Input: part model. Units: mm. Frame: model coordinates. Face numbers are marked on the shaded views. A direction names the side the tool comes from. Round coordinates to 2 decimals unless told otherwise and drop trailing zeros. Order: outer loops, then holes, each group sorted by start corner. A loop starts at its lowest first (then second) coordinate and runs counter-clockwise, first axis right, second up.
Item 1: Cut plane B-B on y = 13. Output: boundary loops of the cut face in (x, z).
Item 2: Cut plane A-A on x = -3. Output: boundary loops of the cut face in (y, z), then the cut area to 3 significant figures.
Item 3: Line query: L1, parallel to Y at x = -22.5, z = -3.35; L2, parallel to Z at x = -17, y = 29; L3, parallel to Y at x = -7, z = -19.25. Output: solid intervals per line, ascending.
Item 4: Cut plane C-C on x = -22.5. Output: boundary loops of the cut face in (y, z).
Item 5: Mould query, pull axis Y, two halves, no side actions, for the marked faces 3, 4 and 5. Classes: released by +Y, released by -Y, zero draft, split by the parting line, or undercut.
Item 6: Reachability of the marked faces 1 and 2 from +Z, -Z, +X, -X, +Y, -Y: full face, straight path, thin tool, end or side. Return the list, or none.
Item 7: First-contact query: pin 1 (3 mm diameter, centred on y = 19.5, z = -4, fed in from +X); pin 2 (8 mm diameter, centred on y = 13, z = -12, fed in from +X). Flat tips, straight axial feed; report the tip coordinate or a pass-through.
Item 8: Cut plane D-D on y = 22. Output: boundary loops of the cut face in (x, z).
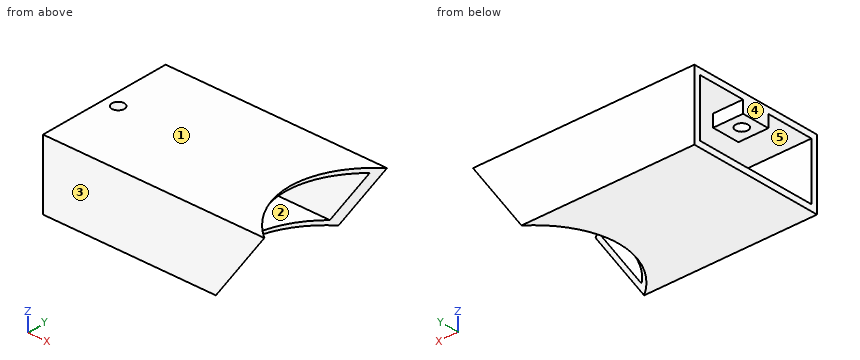
```python
from build123d import *

# Parameters (mm, degrees)
BOSS_EXTRUDE1_DEPTH      = 60
BOSS_EXTRUDE1_DEPTH_BACK = 27
SKETCH1_W                = 22.45
SKETCH1_H                = 43.9
SKETCH1_W_2              = 18.45
SKETCH1_H_2              = 39.9
SKETCH3_W                = 9.697753833
SKETCH3_H                = 9.057928037
SKETCH3_R                = 2
BOSS_EXTRUDE2_DEPTH      = 6
CUT_EXTRUDE1_REACH       = 66.258
SKETCH3_3_R              = 2


with BuildPart() as part:
    # Sketch1 → Boss-Extrude1 (new, two sides: drawn at the far end of the back side and taken through both)
    with BuildSketch(Plane(origin=(0, 0, 0), x_dir=(0, 0, -1), z_dir=(1, 0, 0)).offset(-BOSS_EXTRUDE1_DEPTH_BACK)):
        with Locations((10.58634259, 18.324330998)):
            Rectangle(SKETCH1_W, SKETCH1_H)
        with Locations((10.58634259, 18.324330998)):
            Rectangle(SKETCH1_W_2, SKETCH1_H_2, mode=Mode.SUBTRACT)
    extrude(amount=BOSS_EXTRUDE1_DEPTH + BOSS_EXTRUDE1_DEPTH_BACK)

    # Sketch2 → Cut-Revolve1 (revolve, cut)
    with BuildSketch(Plane(origin=(0, 18.324330998, 0), x_dir=(-1, 0, 0), z_dir=(0, -1, 0))):
        Polygon((-79.85393198, -15.110595304), (-55.279370652, -32.317888394), (-13.19002891, 27.791921119), (-37.764590239, 44.999214209), align=None)
    revolve(axis=Axis((79.85393198, 18.324330998, 15.110595304), (-0.573576436351041, 0, -0.8191520442889954)), mode=Mode.SUBTRACT)

    # Sketch3 → Boss-Extrude2 (add)
    with BuildSketch(Plane.XY.offset(0.63865741)):
        with Locations((-22.151123083, 18.324330997)):
            Rectangle(SKETCH3_W, SKETCH3_H)
        with Locations((-22.5, 18.324330998)):
            Circle(SKETCH3_R, mode=Mode.SUBTRACT)
    extrude(amount=-BOSS_EXTRUDE2_DEPTH)

    # Sketch3<3> → Cut-Extrude1 (cut, up to next)
    with BuildSketch(Plane.XY.offset(0.63865741), mode=Mode.PRIVATE) as cut_extrude1_sk1:
        with Locations((-22.5, 18.324330998)):
            Circle(SKETCH3_3_R)
    cut_extrude1_tool1 = extrude(cut_extrude1_sk1.sketch, amount=-CUT_EXTRUDE1_REACH, mode=Mode.PRIVATE) & part.part
    add(cut_extrude1_tool1.solids().sort_by_distance((-22.5, 18.324331, 0.638657))[0], mode=Mode.SUBTRACT)


solid = part.part
```
From the geometry:
1. outline: (-27, -21.81) - (17.96, -21.81) - (19.36, -19.81) - (-27, -19.81) - close; (-27, -1.36) - (32.28, -1.36) - (33.68, 0.64) - (-27, 0.64) - close
2. outline: (-3.63, -21.81) - (40.27, -21.81) - (40.27, 0.64) - (-3.63, 0.64) - close; hole (-1.63, -19.81) - (38.27, -19.81) - (38.27, -1.36) - (-1.63, -1.36) - close
2. area: 249 mm2
3. L1: y = -3.63 to -1.63, 13.8 to 16.32, 20.32 to 22.85, 38.27 to 40.27
3. L2: z = -21.81 to -19.81, -1.36 to 0.64
3. L3: y = -3.63 to -1.63, 38.27 to 40.27
4. outline: (-3.63, -21.81) - (40.27, -21.81) - (40.27, 0.64) - (20.32, 0.64) - (20.32, -5.36) - (22.85, -5.36) - (22.85, -1.36) - (38.27, -1.36) - (38.27, -19.81) - (-1.63, -19.81) - (-1.63, -1.36) - (13.8, -1.36) - (13.8, -5.36) - (16.32, -5.36) - (16.32, 0.64) - (-3.63, 0.64) - close
5. face 3: released by -Y
5. face 4: zero draft
5. face 5: undercut
6. face 1: +Z, +X, -X, +Y, -Y
6. face 2: +X, -X
7. pin 1: stops at x = -17.3
7. pin 2: passes through
8. outline: (-27, -21.81) - (17.65, -21.81) - (19.05, -19.81) - (-27, -19.81) - close; (-27, -5.36) - (-17.3, -5.36) - (-17.3, -1.36) - (31.97, -1.36) - (33.37, 0.64) - (-27, 0.64) - close
